Geometry check sheet. Reference: drawing and pictorial views, mm from the part's lowest x, y, z. A direction names the side the tool comes from. Coordinates: 2 decimals unless noted, no trailing zeros. Loops run counter-clockwise (first coordinate to the right, second up) from the corner with the lowest first, then second, coordinate; pieces in that order, holes last. Notation, with made-up numbers: (50.5, -9) - (57.5, -9) arc R20 ccw to (57.5, 19) - close; hole circle Ø11 at (75, 78). An arc over 180 degrees is marked (long way). Write each question's results on one line, items separated by ' | '. Start each with the question number.
1. Cross-section at D-D (y = 20). Record the cut outline in (x, z), and give its area (3 significant figures).
2. Cross-section at C-C (z = 26). Record the cut outline in (x, y).
3. Gauge pin test, flat ends, axial feed: P1, Ø2.5, axis at x = 15, y = 21.5, coming from the +Z side; P2, Ø1.2, axis at x = 29.5, z = 17, coming from the +Y side; P3, Ø3.5, axis at x = 23, z = 8, coming from the +Y side. Record the tip position at first contact, or that the pin passes through.
4. Thickness scan on line 1 (X direction, y = 3, z = 27.5); line 2 (Z direction, x = 4, y = 22.75); line 3 (Y direction, x = 5, z = 6.5). Record the ranges inside material, lowest first. Write a range as [from, to].
5. Draft check along X on the marked faces 1, 2 and 3. Enter one of: released by +X, released by -X, zero draft, split by the parting line, or undercut.
6. Tool access check on the marked faces 4, 5 and 6. Record the directions out of +Z, -Z, +X, -X, +Y, -Y that give a thin tool (end or side, any length) a straight path to the whole face; none if there is none.
7. Cross-section at B-B (x = 14). Record the cut outline in (y, z), and give its area (3 significant figures).
8. Cross-section at A-A (y = 7.75). Record the cut outline in (x, z).
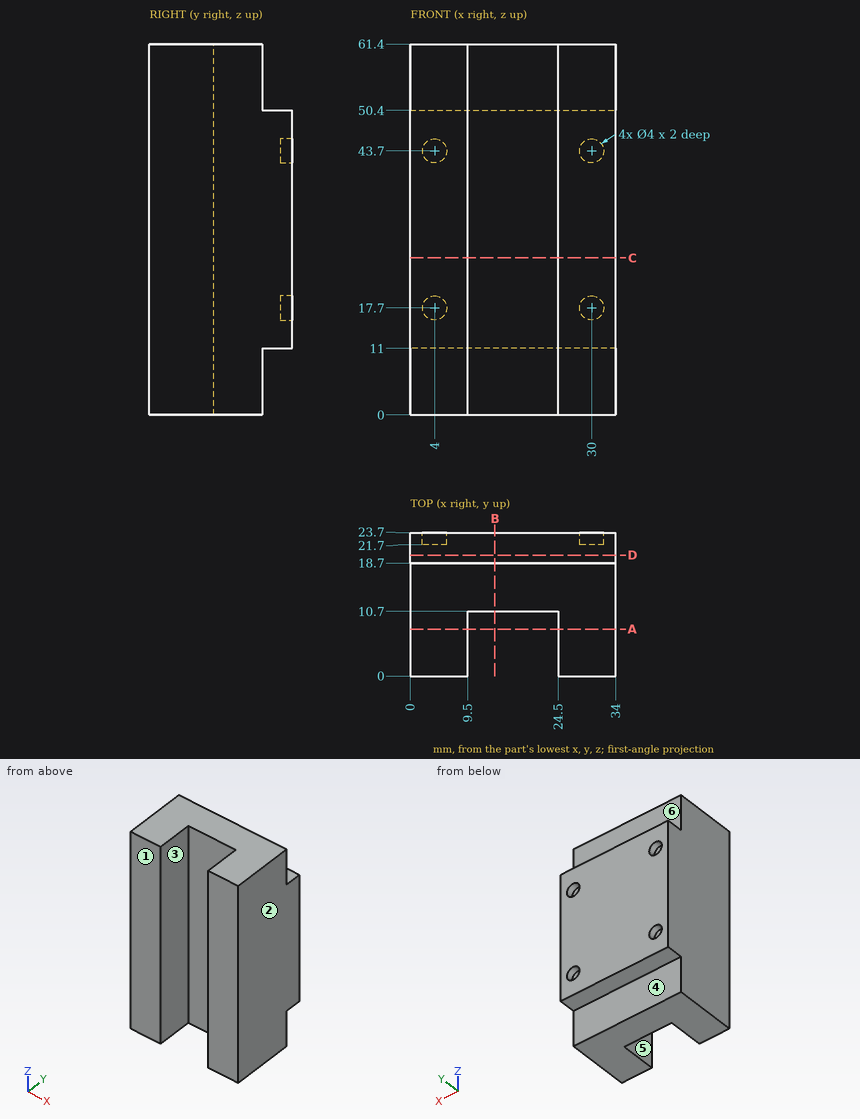
Established:
1) outline: (0, 11) - (34, 11) - (34, 50.4) - (0, 50.4) - close | area: 1,340 mm^2
2) outline: (0, 0) - (9.5, 0) - (9.5, 10.7) - (24.5, 10.7) - (24.5, 0) - (34, 0) - (34, 23.7) - (0, 23.7) - close
3) P1: z = 50.4 | P2: y = 21.7 | P3: y = 18.7
4) line 1: [0, 9.5], [24.5, 34] | line 2: [11, 15.7], [19.7, 41.7], [45.7, 50.4] | line 3: [0, 18.7]
5) face 1: zero draft | face 2: released by +X | face 3: undercut
6) face 4: -Z, +X, -X, +Y | face 5: +Z, -Z, -Y | face 6: +Z, +X, -X, +Y
7) outline: (10.7, 0) - (18.7, 0) - (18.7, 11) - (23.7, 11) - (23.7, 50.4) - (18.7, 50.4) - (18.7, 61.4) - (10.7, 61.4) - close | area: 688 mm^2
8) outline: (0, 0) - (9.5, 0) - (9.5, 61.4) - (0, 61.4) - close; (24.5, 0) - (34, 0) - (34, 61.4) - (24.5, 61.4) - close
